CAD build for the part. Positions are in the model's coordinates, mm. Face numbers are marked on the shaded views. A direction names the side the tool comes from. Give positions to 0.01 mm unless a question says otherwise; leave off trailing zeros. Loops run counter-clockwise (first coordinate to the right, second up) from the corner with the lowest first, then second, coordinate; pieces in that order, holes last. Notation, with made-up numbers: (29, -29.5) -> (72, -29.5) arc R29 ccw to (72, 3.5) -> close; hole circle Ø11 at (27.25, 46). An arc over 180 degrees is marked (long way). Use one line per item in the form item = value.
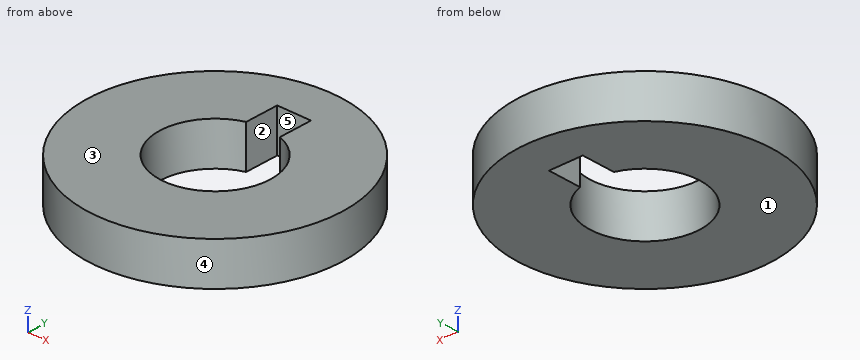
```python
from build123d import *

# Parameters (mm, degrees)
IZIM1_R                     = 15
IZIM1_R_2                   = 6.5
Y_KSEKLIK_EKSTR_ZYON1_DEPTH = 5
IZIM2_W                     = 4
IZIM2_H                     = 4
KES_EKSTR_ZYON1_DEPTH       = 8


with BuildPart() as part:
    # Çizim1 → Yükseklik-Ekstrüzyon1 (new body)
    with BuildSketch(Plane.XY):
        Circle(IZIM1_R)
        Circle(IZIM1_R_2, mode=Mode.SUBTRACT)
    extrude(amount=Y_KSEKLIK_EKSTR_ZYON1_DEPTH)

    # Çizim2 → Kes-Ekstrüzyon1 (cut)
    with BuildSketch(Plane(origin=(0, 0, 0), x_dir=(-1, 0, 0), z_dir=(0, 0, -1))):
        with Locations((0, 8.184658438)):
            Rectangle(IZIM2_W, IZIM2_H)
    extrude(amount=-KES_EKSTR_ZYON1_DEPTH, mode=Mode.SUBTRACT)


solid = part.part
```
1. Tool access for the marked faces 1 and 2: list every direction of +Z, -Z, +X, -X, +Y, -Y with a clear straight run to the whole face (end or side of a thin tool).
Result sheet:
face_1 = -Z, +X, -X, +Y, -Y
face_2 = +Z, -Z
2. Cut at D-D, the plane x = 12. Write the cut outline in (y, z).
Result sheet:
outline = (-9, 0) -> (9, 0) -> (9, 5) -> (-9, 5) -> close
3. Drop flat-ended pins along their axis: P1, Ø1.2, axis at x = -1, z = 3, coming from the -Y side; P2, Ø3, axis at y = 9, z = 3.5, coming from the -X side; P3, Ø1, axis at x = 4, z = 1.5, coming from the -Y side. Give the stop position or say it passes through.
Result sheet:
P1 = -14.99
P2 = -12.99
P3 = -14.59
4. Mould opens along Y. For the marked faces 3, 4 and 5 say: pulls with the +Y half, pulls with the -Y half, needs draft (parallel to the pull), parting line crosses it, or undercut.
Result sheet:
face_3 = needs draft
face_4 = parting line crosses it
face_5 = undercut
5. Cut at B-B, the plane x = 5.25. Write the cut outline in (y, z).
Result sheet:
outline = (-14.05, 0) -> (-3.83, 0) -> (-3.83, 5) -> (-14.05, 5) -> close; (3.83, 0) -> (14.05, 0) -> (14.05, 5) -> (3.83, 5) -> close
6. Drill centre lines: line 1 (Y direction, x = 0, z = 3.1); line 2 (X direction, y = -5.75, z = 2.5); line 3 (X direction, y = -4, z = 4.4). Where is each one in solid material? Low to high.
Result sheet:
line_1 = -15 to -6.5, 10.18 to 15
line_2 = -13.85 to -3.03, 3.03 to 13.85
line_3 = -14.46 to -5.12, 5.12 to 14.46
7. Cut at C-C, the plane z = 0.55. Write the cut outline in (x, y).
Result sheet:
outline = circle Ø30 at (0, 0); hole (-2, 6.18) arc R6.5 ccw (long way) to (2, 6.18) -> (2, 10.18) -> (-2, 10.18) -> close
8. Cut at A-A, the plane y = 0. Write the cut outline in (x, z), then the cut area to 3 significant figures.
Result sheet:
outline = (-15, 0) -> (-6.5, 0) -> (-6.5, 5) -> (-15, 5) -> close; (6.5, 0) -> (15, 0) -> (15, 5) -> (6.5, 5) -> close
area = 85.0 mm^2
